from build123d import *

# Parameters (mm, degrees)
F0_R     = 38.1
F0_R_2   = 29.21
F1_DEPTH = 2.54
F0_R_3   = 25.4
F2_DEPTH = 157.48
F3_R     = 38.1
F3_R_2   = 29.21
F4_DEPTH = 2.54


with BuildPart() as f1:
    # F0 (on Front) → F1 (new body)
    with BuildSketch(Plane.XZ):
        Circle(F0_R)
        Circle(F0_R_2, mode=Mode.SUBTRACT)
    extrude(amount=F1_DEPTH)

    # F0 (on Front) → F2 (join)
    with BuildSketch(Plane.XZ):
        Circle(F0_R_2)
        Circle(F0_R_3, mode=Mode.SUBTRACT)
    extrude(amount=F2_DEPTH)

    # F3 (on face) → F4 (join)
    with BuildSketch(Plane.XZ.offset(157.48)):
        Circle(F3_R)
        Circle(F3_R_2, mode=Mode.SUBTRACT)
    extrude(amount=-F4_DEPTH)


solid = f1.part
Input: part model. Units: mm. Frame: model coordinates. A direction names the side the tool comes from. Round coordinates to 2 decimals unless told otherwise and drop trailing zeros. Loops run counter-clockwise (first coordinate to the right, second up) from the corner with the lowest first, then second, coordinate; pieces in that order, holes last. Notation, with made-up numbers: M 66,-38 L 92,-38 A29 cw 92,-8 Z; hole C 87.25,18 d9. An arc over 180 degrees is marked long. Answer as CSV lines item,"result". Start each with the question number.
(1) First-contact query: pin 1 (4 mm diameter, centred on x = -11.5, y = -126.5, fed in from -Z); pin 2 (4 mm diameter, centred on y = -83.5, z = -22.5, fed in from +X); pin 3 (10 mm diameter, centred on y = -25, z = 7, fed in from +X). Flat tips, straight axial feed; report the tip coordinate or a pass-through.
(2) Reachability of faces 4 (the cylindrical face through (-21.53, -77.67, 19.74)), 5 (the flat face through (8, 0, -25)) from +Z, -Z, +X, -X, +Y, -Y: full face, straight path, thin tool, end or side. Return the list, or none.
(3) Section B-B, the plane x = 0. Output: boundary loops of the cut face in (y, z), plus the area to 3 significant figures.
(4) Section C-C, the plane y = -52.5. Output: boundary loops of the cut face in (x, z), plus the area to 3 significant figures.
(5) Line query: line 1 (Z direction, x = 0, y = -91); line 2 (Y direction, x = 1, z = 32.5); line 3 (X direction, y = -12, z = 4.5). Output: solid intervals per line, ascending. Write a range as [from, to].
(6) Section A-A, the plane z = 0. Output: boundary loops of the cut face in (x, y), plus the area to 3 significant figures.
(7) Draft query along Z for faces 1 (the cylindrical face through (-30.235, -156.228, -23.183)), 2 (the cylindrical face through (-5.506, -77.638, -24.796)), 3 (the flat face through (8, -157.48, -25)). Return one class per face: released by +Z, released by -Z, zero draft, split by the parting line, or undercut.
Values found:
1,pin 1,"stops at z = -27.62"
1,pin 2,"stops at x = 20.81"
1,pin 3,"stops at x = 29.14"
2,face 4,"none"
2,face 5,"+Z, -Z, +X, -X, +Y"
3,outline,"M -157.48,-38.1 L -154.94,-38.1 L -154.94,-29.21 L -2.54,-29.21 L -2.54,-38.1 L 0,-38.1 L 0,-25.4 L -157.48,-25.4 Z; M -157.48,25.4 L 0,25.4 L 0,38.1 L -2.54,38.1 L -2.54,29.21 L -154.94,29.21 L -154.94,38.1 L -157.48,38.1 Z"
3,area,"1,290 mm²"
4,outline,"C 0,0 d58.42; hole C 0,0 d50.8"
4,area,"654 mm²"
5,line 1,"z = [-29.21, -25.4], [25.4, 29.21]"
5,line 2,"y = [-157.48, -154.94], [-2.54, 0]"
5,line 3,"x = [-28.86, -25], [25, 28.86]"
6,outline,"M -38.1,-157.48 L -25.4,-157.48 L -25.4,0 L -38.1,0 L -38.1,-2.54 L -29.21,-2.54 L -29.21,-154.94 L -38.1,-154.94 Z; M 25.4,-157.48 L 38.1,-157.48 L 38.1,-154.94 L 29.21,-154.94 L 29.21,-2.54 L 38.1,-2.54 L 38.1,0 L 25.4,0 Z"
6,area,"1,290 mm²"
7,face 1,"split by the parting line"
7,face 2,"undercut"
7,face 3,"zero draft"
